```python
from build123d import *

# Parameters (mm, degrees)
SKETCH1_R           = 1.5
BOSS_EXTRUDE1_DEPTH = 4.15
BOSS_EXTRUDE2_DEPTH = 2
SKETCH3_R           = 1.5
BOSS_EXTRUDE3_DEPTH = 4.15
SKETCH4_R           = 1
CUT_EXTRUDE1_DEPTH  = 38.560917188


with BuildPart() as part:
    # Sketch1 → Boss-Extrude1 (new body)
    with BuildSketch(Plane(origin=(0, 0, 0), x_dir=(1, 0, 0), z_dir=(0, 1, 0))):
        with Locations(Location((0, 0, 0), (0, 0, 90))):
            Circle(SKETCH1_R)
    extrude(amount=BOSS_EXTRUDE1_DEPTH)

    # Sketch2 → Boss-Extrude2 (add)
    with BuildSketch(Plane(origin=(0, 4.15, 0), x_dir=(1, 0, 0), z_dir=(0, 1, 0))):
        with BuildLine():
            Line((35, 2), (0, 2))
            ThreePointArc((0, 2), (-2, 0), (0, -2))
            Line((0, -2), (35, -2))
            ThreePointArc((35, -2), (37, 0), (35, 2))
        make_face()
    extrude(amount=BOSS_EXTRUDE2_DEPTH)

    # Sketch3 → Boss-Extrude3 (add)
    with BuildSketch(Plane.XZ.offset(-4.15)):
        with Locations(Location((35, 0, 0), (0, 0, 90))):
            Circle(SKETCH3_R)
    extrude(amount=BOSS_EXTRUDE3_DEPTH)

    # Sketch4 → Cut-Extrude1 (cut, through all)
    with BuildSketch(Plane(origin=(0, 6.15, 0), x_dir=(1, 0, 0), z_dir=(0, 1, 0))):
        with Locations(Location((0, 0, 0), (0, 0, 270))):
            Circle(SKETCH4_R)
        with Locations(Location((35, 0, 0), (0, 0, 270))):
            Circle(SKETCH4_R)
    extrude(amount=-CUT_EXTRUDE1_DEPTH, mode=Mode.SUBTRACT)


solid = part.part
```
Check sheet for the modelled part. Datum: model origin and axes. Units: mm. A direction names the side the tool comes from. Coordinates: 2 decimals unless noted, no trailing zeros. Loops run counter-clockwise (first coordinate to the right, second up) from the corner with the lowest first, then second, coordinate; pieces in that order, holes last.
1) Sectioned sample at D-D (x = 19.5). Record the boundary of the cut face in (y, z), and give its area (3 significant figures).
2) Material ranges on probe 1 along X at (y, z) = (3.75, 0); probe 2 along X at (y, z) = (5.5, 0.05); probe 3 along X at (y, z) = (4, -0.9), recorded low to high.
3) Gauge pin test, flat ends, axial feed: pin 1 (1.8 mm diameter, centred on x = 35, z = 0, fed in from -Y); pin 2 (2 mm diameter, centred on x = 8, z = -1, fed in from -Y). Record the tip position at first contact, or that the pin passes through.
4) Sectioned sample at C-C (y = 5). Record the boundary of the cut face in (x, z).
5) Release check for a two-part mould opening along X. For faces 3 (the face through (36, 3, 0)), 4 (the face through (-1, 3, 0)), 5 (the face through (18, 5, -2)), 6 (the face through (37, 5, 0)) record: released by +X, released by -X, zero draft, split by the parting line, or undercut.
6) Sectioned sample at A-A (z = 0). Record the boundary of the cut face in (x, y).
7) Sectioned sample at B-B (y = 0.75). Record the boundary of the cut face in (x, z).
8) Access from +Z, -Z, +X, -X, +Y, -Y to the whole of each face (thin tool, end or side, straight path). Record for faces 1 (the face through (36.464, 2.104, -0.325)), 2 (the face through (17, 5, 2)).
Check sheet entries:
1. outline: (4.15, -2) - (6.15, -2) - (6.15, 2) - (4.15, 2) - close
1. area: 8.00 mm2
2. probe 1: x = -1.5 to -1, 1 to 1.5, 33.5 to 34, 36 to 36.5
2. probe 2: x = -2 to -1, 1 to 34, 36 to 37
2. probe 3: x = -1.2 to -0.44, 0.44 to 1.2, 33.8 to 34.56, 35.44 to 36.2
3. pin 1: passes through
3. pin 2: stops at y = 4.15
4. outline: (0, -2) - (35, -2) arc R2 ccw to (35, 2) - (0, 2) arc R2 ccw to start; hole circle Ø2 at (0, 0); hole circle Ø2 at (35, 0)
5. face 3: undercut
5. face 4: undercut
5. face 5: zero draft
5. face 6: released by +X
6. outline: (-2, 4.15) - (-1.5, 4.15) - (-1.5, 0) - (-1, 0) - (-1, 6.15) - (-2, 6.15) - close; (1, 0) - (1.5, 0) - (1.5, 4.15) - (33.5, 4.15) - (33.5, 0) - (34, 0) - (34, 6.15) - (1, 6.15) - close; (36, 0) - (36.5, 0) - (36.5, 4.15) - (37, 4.15) - (37, 6.15) - (36, 6.15) - close
7. outline: circle Ø3 at (0, 0); circle Ø3 at (35, 0); hole circle Ø2 at (0, 0); hole circle Ø2 at (35, 0)
8. face 1: -Y
8. face 2: +Z, +X, -X, +Y, -Y
